For this review, use the dimensioned drawing (mm, ordinates from the lowest corner) and the shaded views. Give positions to 0.01 mm unless a question says otherwise; leave off trailing zeros. Order: outer loops, then holes, each group sorted by start corner. A loop starts at its lowest first (then second) coordinate and runs counter-clockwise, first axis right, second up. Notation, with made-up numbers: (39, 73.25) -> (81, 73.25) arc R32 ccw to (81, 111.25) -> close; hole circle Ø4 at (0.5, 51). An arc over 180 degrees is marked (long way). Answer as a JSON object with one key per item and string values. Group by question number.
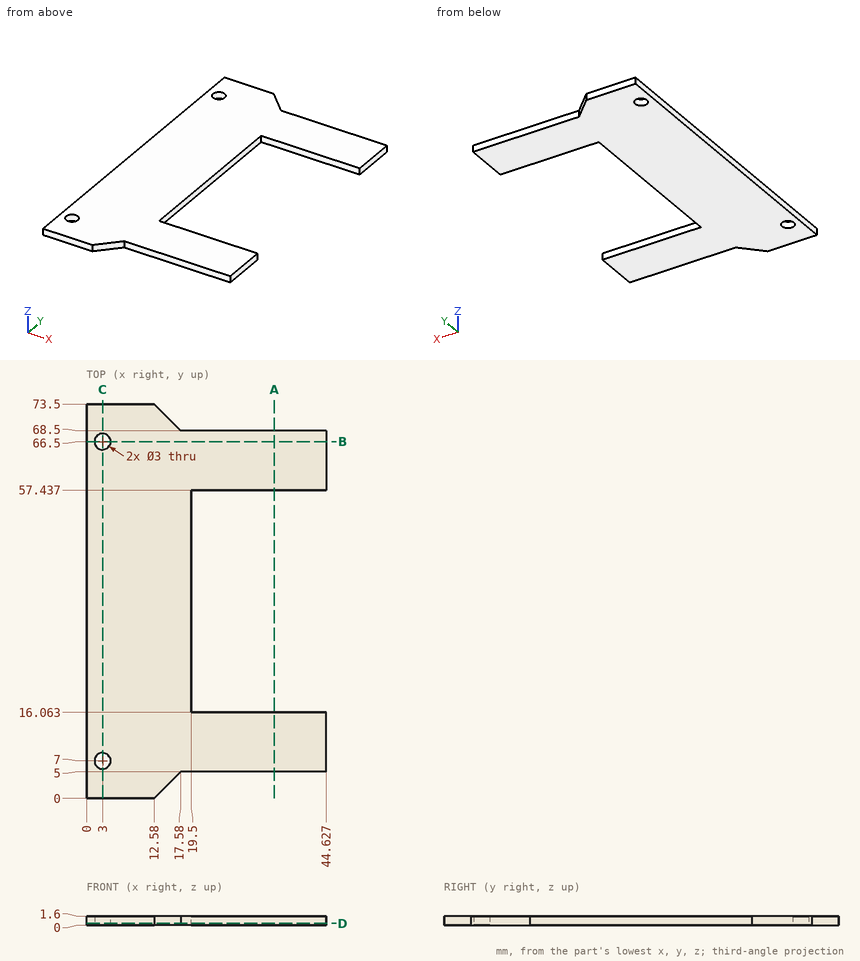
1. Take a section at D-D on z = 0.3. Give the boundary of the cut face in (x, y).
2. Take a section at A-A on x = 35. Give the boundary of the cut face in (y, z), plus the area to 3 significant figures.
3. Take a section at C-C on x = 3. Give the boundary of the cut face in (y, z), plus the area to 3 significant figures.
4. For probe 1 along Y at (x, z) = (3, 1); probe 2 along X at (y, z) = (66.5, 1.05); probe 3 along Y at (x, z) = (29, 0.8), list the stretches that pass through material, from the lowest coordinate up. Write a range as [from, to].
5. For pin 1 (0.8 mm diameter, centred on x = 30, z = 1, fed in from -Y); pin 2 (0.8 mm diameter, centred on y = 35.5, z = 0.5, fed in from +X), all flat-tipped, find the tip position at first contact; note any pin that passes through.
6. Take a section at B-B on y = 66.5. Give the boundary of the cut face in (x, z).
Checks:
{
 "1": {"outline": "(0, 0) -> (12.58, 0) -> (17.58, 5) -> (44.63, 5) -> (44.63, 16.06) -> (19.5, 16.06) -> (19.5, 57.44) -> (44.63, 57.44) -> (44.63, 68.5) -> (17.58, 68.5) -> (12.58, 73.5) -> (0, 73.5) -> close; hole circle Ø3 at (3, 7); hole circle Ø3 at (3, 66.5)"},
 "2": {"outline": "(5, 0) -> (16.06, 0) -> (16.06, 1.6) -> (5, 1.6) -> close; (57.44, 0) -> (68.5, 0) -> (68.5, 1.6) -> (57.44, 1.6) -> close", "area": "35.4 mm2"},
 "3": {"outline": "(0, 0) -> (5.5, 0) -> (5.5, 1.6) -> (0, 1.6) -> close; (8.5, 0) -> (65, 0) -> (65, 1.6) -> (8.5, 1.6) -> close; (68, 0) -> (73.5, 0) -> (73.5, 1.6) -> (68, 1.6) -> close", "area": "108 mm2"},
 "4": {"probe 1": "y = [0, 5.5], [8.5, 65], [68, 73.5]", "probe 2": "x = [0, 1.5], [4.5, 44.63]", "probe 3": "y = [5, 16.06], [57.44, 68.5]"},
 "5": {"pin 1": "stops at y = 5", "pin 2": "stops at x = 19.5"},
 "6": {"outline": "(0, 0) -> (1.5, 0) -> (1.5, 1.6) -> (0, 1.6) -> close; (4.5, 0) -> (44.63, 0) -> (44.63, 1.6) -> (4.5, 1.6) -> close"}
}
